```python
from build123d import *

# Parameters (mm, degrees)
BOSS_EXTRUDE1_DEPTH     = 5
SKETCH2_R               = 1.9
BOSS_EXTRUDE2_DEPTH     = 9.8
CUT_EXTRUDE2_DEPTH      = 1
CUT_EXTRUDE2_DEPTH_BACK = 1
FILLET1_R               = 1
FILLET2_R               = 0.8


with BuildPart() as part:
    # Sketch1 → Boss-Extrude1 (new body)
    with BuildSketch(Plane(origin=(0, 0, 0), x_dir=(1, 0, 0), z_dir=(0, 1, 0))):
        with BuildLine():
            Line((-3.9, 3.9), (0, 3.9))
            ThreePointArc((0, 3.9), (2.757716447, 2.757716447), (3.9, 0))
            Line((3.9, 0), (3.9, -3.9))
            Line((3.9, -3.9), (0, -3.9))
            ThreePointArc((0, -3.9), (-2.757716447, -2.757716447), (-3.9, 0))
            Line((-3.9, 0), (-3.9, 3.9))
        make_face()
    extrude(amount=BOSS_EXTRUDE1_DEPTH)

    # Sketch2 → Boss-Extrude2 (add)
    with BuildSketch(Plane(origin=(0, 5, 0), x_dir=(1, 0, 0), z_dir=(0, 1, 0))):
        with Locations(Location((0, 0, 0), (0, 0, 270))):
            Circle(SKETCH2_R)
    extrude(amount=BOSS_EXTRUDE2_DEPTH)

    # Sketch3 → Cut-Extrude2 (cut, two sides: drawn at the far end of the back side and taken through both)
    with BuildSketch(Plane(origin=(0, 2.5, 0), x_dir=(1, 0, 0), z_dir=(0, 1, 0)).offset(-CUT_EXTRUDE2_DEPTH_BACK)):
        with BuildLine():
            Line((-3.9, 0), (-3.9, 3.9))
            Line((-3.9, 3.9), (0, 3.9))
            ThreePointArc((0, 3.9), (2.757716447, 2.757716447), (3.9, 0))
            Line((3.9, 0), (3.9, -3.9))
            Line((3.9, -3.9), (0, -3.9))
            ThreePointArc((0, -3.9), (-2.757716447, -2.757716447), (-3.9, 0))
        make_face()
        with BuildLine():
            Line((-2.9, 0), (-2.9, 2.9))
            Line((-2.9, 2.9), (0, 2.9))
            ThreePointArc((0, 2.9), (2.050609665, 2.050609665), (2.9, 0))
            Line((2.9, 0), (2.9, -2.9))
            Line((2.9, -2.9), (0, -2.9))
            ThreePointArc((0, -2.9), (-2.050609665, -2.050609665), (-2.9, 0))
        make_face(mode=Mode.SUBTRACT)
    extrude(amount=CUT_EXTRUDE2_DEPTH + CUT_EXTRUDE2_DEPTH_BACK, mode=Mode.SUBTRACT)

    # Fillet1
    fillet1_edges = [part.edges().sort_by_distance(p)[0] for p in [
        (2.9, 3.5, 1.45),
        (2.050609665, 3.5, -2.050609665),
        (1.45, 3.5, 2.9),
        (-2.050609665, 3.5, 2.050609665),
        (2.9, 1.5, 1.45),
        (2.050609665, 1.5, -2.050609665),
        (-2.9, 1.5, -1.45),
        (1.45, 1.5, 2.9),
        (-1.45, 3.5, -2.9),
        (-2.9, 3.5, -1.45),
        (-1.45, 1.5, -2.9),
        (-2.050609665, 1.5, 2.050609665),
    ]]
    fillet(fillet1_edges, radius=FILLET1_R - 0.0001)  # a hair under: the kernel refuses the full size

    # Fillet2
    fillet2_edges = [part.edges().sort_by_distance(p)[0] for p in [
        (0, 14.8, -1.9),
    ]]
    fillet(fillet2_edges, radius=FILLET2_R)


solid = part.part
```
Input: part model. Units: mm. Frame: model coordinates. A direction names the side the tool comes from. Coordinates: 2 decimals unless noted, no trailing zeros. Loops run counter-clockwise (first coordinate to the right, second up) from the corner with the lowest first, then second, coordinate; pieces in that order, holes last. Notation, with made-up numbers: (43, 5.25) -> (78, 5.25) arc R24 ccw to (78, 37.25) -> close; hole circle Ø6 at (-7.5, 12). An arc over 180 degrees is marked (long way). Use a Markdown table: item, result.
1) Cut plane A-A (y = 4.5). Return the cut outline in (x, z), then the cut area to 3 significant figures.
Results found:
| item | result |
|---|---|
| outline | (-3.9, -3.9) -> (0, -3.9) arc R3.9 ccw to (3.9, 0) -> (3.9, 3.9) -> (0, 3.9) arc R3.9 ccw to (-3.9, 0) -> close |
| area | 54.3 mm2 |
2) Cut plane B-B (y = 7). Return the cut outline in (x, z), then the cut area to 3 significant figures.
Results found:
| item | result |
|---|---|
| outline | circle Ø3.8 at (0, 0) |
| area | 11.3 mm2 |
3) Contact query for a flat-ended pin moving along its axis: pin 1 (2 mm diameter, centred on x = -0.5, y = 10.5, fed in from +Z). Output: stop coordinate, or through.
Results found:
| item | result |
|---|---|
| pin 1 | stops at z = 1.9 |
4) Access query for faces 1 (the cylindrical face through (-1.489, 3.199, -3.185)), 2 (the cylindrical face through (3.185, 3.199, 1.544)), 3 (the cylindrical face through (-0.728, 9.437, 1.755)). Directions: +Z, -Z, +X, -X, +Y, -Y. A direction counts if a zero-diameter tool reaches every point of the face in a straight line with its end or side. Return the directions, or none.
Results found:
| item | result |
|---|---|
| face 1 | -Z, +X, -X |
| face 2 | +Z, -Z, +X |
| face 3 | +Y |
5) Cut plane C-C (y = 1.75). Return the cut outline in (x, z), then the cut area to 4 significant figures.
Results found:
| item | result |
|---|---|
| outline | (-3.24, -3.24) -> (0, -3.24) arc R3.24 ccw to (3.24, 0) -> (3.24, 3.24) -> (0, 3.24) arc R3.24 ccw to (-3.24, 0) -> close |
| area | 37.45 mm2 |
6) Material intervals for line 1 along Y through (x, z) = (-3, -1.25); line 2 along Y through (x, z) = (-1.75, -2.5); line 3 along Y through (x, z) = (-2.75, 1.25), sorted ascending. Write a range as from..to.
Results found:
| item | result |
|---|---|
| line 1 | y = 0..2.06, 2.94..5 |
| line 2 | y = 0..5 |
| line 3 | y = 0..2.02, 2.98..5 |
